from build123d import *

# Parameters (mm, degrees)
SKETCH2_R           = 12.7
SKETCH4_R           = 12.7
BOSS_EXTRUDE2_DEPTH = 1528.8


with BuildPart() as part:
    # Sweep1: sweep along a path in Sketch1
    with BuildLine(Plane.XY) as sweep1_path:
        Line((0, 0), (0, 300))
        ThreePointArc((0, 300), (37.197438789, 389.802561211), (127, 427))
        Line((127, 427), (1397, 427))
        ThreePointArc((1397, 427), (1486.802561211, 389.802561211), (1524, 300))
        Line((1524, 300), (1524, 0))
    # Sketch2 → Sweep1 (sweep)
    with BuildSketch(Plane(origin=(0, 0, 0), x_dir=(1, 0, 0), z_dir=(0, 1, 0))):
        Circle(SKETCH2_R)
    sweep(path=sweep1_path.line)

    # Sketch4 → Boss-Extrude2 (add)
    with BuildSketch(Plane(origin=(0, 0, 0), x_dir=(0, 0, -1), z_dir=(1, 0, 0))):
        with Locations((0, 300)):
            Circle(SKETCH4_R)
    extrude(amount=BOSS_EXTRUDE2_DEPTH)


solid = part.part
Source: CAD feature listing. Evaluate the final solid. Frame: model axes, mm. A direction names the side the tool comes from. Coordinates: 2 decimals unless noted, no trailing zeros. Order: outer loops, then holes, each group sorted by start corner. A loop starts at its lowest first (then second) coordinate and runs counter-clockwise, first axis right, second up. Notation, with made-up numbers: M -26.5,-26 L 10.5,-26 A34 ccw 10.5,13 Z; hole C 35,-13.75 d2. An arc over 180 degrees is marked long. Write each question's results on one line, items separated by ' | '. Start each with the question number.
Item 1: First-contact query: pin 1 Ø5 at (y, z) = (391, -6) entering from -X; pin 2 Ø4 at (y, z) = (79.5, 9.5) entering from -X; pin 3 Ø12 at (x, z) = (1266, -5) entering from -Y. Flat tips, straight axial feed; report the tip coordinate or a pass-through.
Item 2: Cut plane B-B (y = 135). Return loops of the section in (x, z).
Item 3: Cut plane C-C (x = 1117). Return loops of the section in (y, z), and give its area (3 significant figures).
Item 4: Draft query along X for faces 4 (the face through (0, 0, 0)), 5 (the face through (1511.886, 147.9, -3.815)). Return one class per face: pulls with the +X half, pulls with the -X half, needs draft (parallel to the pull), parting line crosses it, or undercut.
Item 5: Line query: probe 1 along X at (y, z) = (107.5, 0); probe 2 along Y at (x, z) = (1114.5, 1.75); probe 3 along X at (y, z) = (56, -2.75). Output: solid intervals per line, ascending.
Item 6: Set-up query: faces 1 (the face through (1524, 0, 0)), 2 (the face through (6.827, 152.1, -10.709)), 3 (the face through (770.89, 414.886, -3.815)). Return all of +Z, -Z, +X, -X, +Y, -Y with unobstructed straight access to the full face (end or side cutting, diameter ignored); none if empty.
Item 7: Cut plane A-A (z = 6.75). Return loops of the section in (x, y).
Checked values:
1) pin 1: stops at x = 20.38 | pin 2: stops at x = -10.25 | pin 3: stops at y = 287.3
2) outline: C 0,0 d25.4; C 1524,0 d25.4
3) outline: C 300,0 d25.4; C 427,0 d25.4 | area: 1,010 mm2
4) face 4: needs draft | face 5: undercut
5) probe 1: x = -12.7 to 12.7, 1511.3 to 1536.7 | probe 2: y = 287.42 to 312.58, 414.42 to 439.58 | probe 3: x = -12.4 to 12.4, 1511.6 to 1536.4
6) face 1: +Z, -Z, +X, -X, -Y | face 2: -Y | face 3: none
7) outline: M -10.76,0 L 10.76,0 L 10.76,289.24 L 1513.24,289.24 L 1513.24,0 L 1534.76,0 L 1534.76,300 A137.76 ccw 1397,437.76 L 127,437.76 A137.76 ccw -10.76,300 Z; hole M 11.26,310.76 L 1512.74,310.76 A116.24 ccw 1397,416.24 L 127,416.24 A116.24 ccw Z
